For this review, take the finished solid that the model builds, in its own axes (mm). A direction names the side the tool comes from. Round coordinates to 2 decimals unless told otherwise and drop trailing zeros. Order: outer loops, then holes, each group sorted by start corner. A loop starts at its lowest first (then second) coordinate and runs counter-clockwise, first axis right, second up. Notation, with made-up numbers: M 87,53 L 130,53 A5 ccw 130,59 Z; hole C -34.5,18.25 d6. An arc over 180 degrees is marked long. Write item = value, one per line. Start each with the question number.
from build123d import *

# Parameters (mm, degrees)
ESQUISSE1_W             = 31.7
ESQUISSE1_H             = 43.35
BOSS_EXTRU_1_DEPTH      = 2
ESQUISSE2_W             = 54.15
ESQUISSE2_H             = 52.075
ESQUISSE2_W_2           = 34.15
ESQUISSE2_H_2           = 46.15
BOSS_EXTRU_2_DEPTH      = 3
ENL_V_MAT_EXTRU_1_DEPTH = 6
CONG_1_R                = 10
ESQUISSE4_R             = 1.1
ESQUISSE4_W             = 2
ESQUISSE4_H             = 20.22
ESQUISSE4_W_2           = 2.219999677
ESQUISSE4_H_2           = 20.218803133
BOSS_EXTRU_3_DEPTH      = 5
CONG_2_R                = 1
CONG_3_R                = 5
ESQUISSE5_R             = 9.6
ENL_V_MAT_EXTRU_2_DEPTH = 6
ESQUISSE7_W             = 31.7
ESQUISSE7_H             = 43.35
ENL_V_MAT_EXTRU_3_DEPTH = 6
ESQUISSE7_4_W           = 34.15
ESQUISSE7_4_H           = 46.15
ENL_V_MAT_EXTRU_4_DEPTH = 3


with BuildPart() as part:
    # Esquisse1 → Boss.-Extru.1 (new body)
    with BuildSketch(Plane.XY):
        Polygon((-20.243056538, 24.478190482), (-20.243056538, -25.521809518), (-20.243056538, -25.596809518), (6.831943462, -25.596809518), (33.906943462, -25.596809518), (33.906943462, -25.521809518), (33.906943462, 24.478190482), (33.906943462, 26.478190482), (5.831943462, 26.478190482), (-20.243056538, 26.478190482), align=None)
        with Locations((6.356943462, -0.426809518)):
            Rectangle(ESQUISSE1_W, ESQUISSE1_H, mode=Mode.SUBTRACT)
    extrude(amount=BOSS_EXTRU_1_DEPTH)

    # Esquisse2 → Boss.-Extru.2 (add)
    with BuildSketch(Plane.XY.offset(2)):
        with Locations((6.831943462, 0.440690482)):
            Rectangle(ESQUISSE2_W, ESQUISSE2_H)
        with Locations((5.881943462, -0.331809518)):
            Rectangle(ESQUISSE2_W_2, ESQUISSE2_H_2, mode=Mode.SUBTRACT)
    extrude(amount=BOSS_EXTRU_2_DEPTH)

    # Esquisse3 → Enl_v. mat.-Extru.1 (cut, through all)
    with BuildSketch(Plane.XY.offset(5)):
        Polygon((-17.730491461, -9.839116901), (-17.730491461, 10.380883099), (-15.510491784, 10.379686232), (-15.730491461, -9.839116901), align=None)
        Polygon((28.519508539, -9.839116901), (28.299508862, 10.379686232), (30.519508539, 10.380883099), (30.519508539, -9.839116901), align=None)
    extrude(amount=-ENL_V_MAT_EXTRU_1_DEPTH, mode=Mode.SUBTRACT)

    # Cong_1
    cong_1_edges = [part.edges().sort_by_distance(p)[0] for p in [
        (-20.243056538, 26.478190482, 2.5),
        (33.906943462, 26.478190482, 2.5),
        (33.906943462, -25.596809518, 2.5),
        (-20.243056538, -25.596809518, 2.5),
    ]]
    fillet(cong_1_edges, radius=CONG_1_R)

    # Esquisse4 → Boss.-Extru.3 (add)
    with BuildSketch(Plane.XY):
        with BuildLine():
            Line((-9.068056538, 38.678190482), (-4.418056538, 38.678190482))
            Line((-4.418056538, 38.678190482), (-4.418056538, 26.478190482))
            Line((-4.418056538, 26.478190482), (18.081943462, 26.478190482))
            Line((18.081943462, 26.478190482), (18.081943462, 38.678190482))
            Line((18.081943462, 38.678190482), (22.731943462, 38.678190482))
            ThreePointArc((22.731943462, 38.678190482), (30.955617573, 28.905183532), (33.906943462, 16.478190482))
            Line((33.906943462, 16.478190482), (33.906943462, -15.596809518))
            ThreePointArc((33.906943462, -15.596809518), (30.978011273, -22.66787733), (23.906943462, -25.596809518))
            Line((23.906943462, -25.596809518), (19.895450173, -31.759659919))
            ThreePointArc((19.895450173, -31.759659919), (7.395450173, -44.259659919), (-5.104549827, -31.759659919))
            Line((-5.104549827, -31.759659919), (-10.243056538, -25.596809518))
            ThreePointArc((-10.243056538, -25.596809518), (-17.31412435, -22.66787733), (-20.243056538, -15.596809518))
            Line((-20.243056538, -15.596809518), (-20.243056538, 16.478190482))
            ThreePointArc((-20.243056538, 16.478190482), (-17.29173065, 28.905183532), (-9.068056538, 38.678190482))
        make_face()
        with Locations((-6.743056538, 32.578190482)):
            Circle(ESQUISSE4_R, mode=Mode.SUBTRACT)
        with Locations((20.406943462, 32.578190482)):
            Circle(ESQUISSE4_R, mode=Mode.SUBTRACT)
        with Locations((-16.730491461, 0.270883099)):
            Rectangle(ESQUISSE4_W, ESQUISSE4_H, mode=Mode.SUBTRACT)
        with Locations((29.409508701, 0.270284666)):
            Rectangle(ESQUISSE4_W_2, ESQUISSE4_H_2, mode=Mode.SUBTRACT)
    extrude(amount=BOSS_EXTRU_3_DEPTH)

    # Cong_2
    cong_2_edges = [part.edges().sort_by_distance(p)[0] for p in [
        (-9.068056538, 38.678190482, 2.5),
        (22.731943462, 38.678190482, 2.5),
        (18.081943462, 38.678190482, 2.5),
        (18.081943462, 26.478190482, 2.5),
        (-4.418056538, 26.478190482, 2.5),
        (-4.418056538, 38.678190482, 2.5),
    ]]
    fillet(cong_2_edges, radius=CONG_2_R)

    # Cong_3
    cong_3_edges = [part.edges().sort_by_distance(p)[0] for p in [
        (-10.243056538, -25.596809518, 2.5),
        (23.906943462, -25.596809518, 2.5),
    ]]
    fillet(cong_3_edges, radius=CONG_3_R)

    # Esquisse5 → Enl_v. mat.-Extru.2 (cut, through all)
    with BuildSketch(Plane.XY.offset(5)):
        with Locations((7.395450173, -31.759659919)):
            Circle(ESQUISSE5_R)
    extrude(amount=-ENL_V_MAT_EXTRU_2_DEPTH, mode=Mode.SUBTRACT)

    # Esquisse7 → Enl_v. mat.-Extru.3 (cut, through all)
    with BuildSketch(Plane.XY.offset(5)):
        with Locations((6.356943462, 2.63695892)):
            Rectangle(ESQUISSE7_W, ESQUISSE7_H)
    extrude(amount=-ENL_V_MAT_EXTRU_3_DEPTH, mode=Mode.SUBTRACT)

    # Esquisse7_4 → Enl_v. mat.-Extru.4 (cut)
    with BuildSketch(Plane.XY.offset(5)):
        with Locations((6.831943462, 2.54195892)):
            Rectangle(ESQUISSE7_4_W, ESQUISSE7_4_H)
    extrude(amount=-ENL_V_MAT_EXTRU_4_DEPTH, mode=Mode.SUBTRACT)


solid = part.part
(1) For faces 1 (the flat face through (25, -2, 5)), 2 (the flat face through (-4.418, 33, 2)), 3 (the flat face through (29, 10.38, 2)), list the 3-axis set-ups (+Z, -Z, +X, -X, +Y, -Y) from which the entire face can be reached by the end or side of a thin tool; tool diameter is ignored.
(2) We need section B-B, the plane x = -0.5. Write out the cut boundary in (y, z), then the cut area to 3 significant figures.
(3) For line 1 along X through (y, z) = (10, 0.95); line 2 along X through (y, z) = (-14, 3.2); line 3 along X through (y, z) = (-3, 1), list the stretches that pass through material, from the lowest coordinate up.
(4) Insertion check: pin 1 (1.6 mm diameter, centred on x = 29.5, z = 3, fed in from +Y); pin 2 (1 mm diameter, centred on x = 4.5, z = 1, fed in from +Y); pin 3 (5 mm diameter, centred on x = -4, y = -15.5, fed in from +Z); pin 4 (0.6 mm diameter, centred on x = -16.5, z = 3.5, fed in from +Y). Each pin has a flat end and moves straight along its axis. Give the tip position at first contact, or say it passes through.
(5) We need section D-D, the plane z = 3.55. State how many separate pieces and enclosed holes the cut face has, then the cut area to 3 significant figures.
(6) Draft analysis for pull direction X (two halves, no side actions). For faces 4 (the flat face through (-10, 3, 2)), 5 (the flat face through (-20.243, 0, 2)), 6 (the flat face through (-7, 38.678, 2)), state which applies: released by +X, released by -X, zero draft, split by the parting line, or undercut.
(7) We need section A-A, the plane y = -11. Write out the cut boundary in (x, z).
(8) We need section C-C, the plane y = 1. Write out the cut boundary in (x, z).
Values:
q1.face_1 = +Z, +X, -X, +Y, -Y
q1.face_2 = +Z, -Z, +Y
q1.face_3 = +Z, -Z
q2.outline = M -41.45,0 L -37.22,0 L -37.22,5 L -41.45,5 Z; M -26.3,0 L -19.04,0 L -19.04,2 L -20.53,2 L -20.53,5 L -26.3,5 Z; M 24.31,0 L 26.48,0 L 26.48,5 L 25.62,5 L 25.62,2 L 24.31,2 Z
q2.area = 59.9 mm²
q3.line_1 = -20.24 to -17.73, -15.73 to -9.49, 22.21 to 28.3, 30.52 to 33.91
q3.line_2 = -20.24 to -10.24, 23.91 to 33.91
q3.line_3 = -20.24 to -17.73, -15.73 to -9.49, 22.21 to 28.45, 30.52 to 33.91
q4.pin_1 = 32.62
q4.pin_2 = 26.48
q4.pin_3 = through
q4.pin_4 = 30.87
q5.separate_pieces = 1
q5.enclosed_holes = 6
q5.area = 1,490 mm²
q6.face_4 = undercut
q6.face_5 = released by -X
q6.face_6 = zero draft
q7.outline = M -20.24,0 L -9.49,0 L -9.49,2 L -10.24,2 L -10.24,5 L -20.24,5 Z; M 22.21,0 L 33.91,0 L 33.91,5 L 23.91,5 L 23.91,2 L 22.21,2 Z
q8.outline = M -20.24,0 L -17.73,0 L -17.73,5 L -20.24,5 Z; M -15.73,0 L -9.49,0 L -9.49,2 L -10.24,2 L -10.24,5 L -15.73,5 Z; M 22.21,0 L 28.4,0 L 28.4,5 L 23.91,5 L 23.91,2 L 22.21,2 Z; M 30.52,0 L 33.91,0 L 33.91,5 L 30.52,5 Z
